Autodesk Inventor part; units mm, degrees
ref_plane "YZ Plane" through (0, 0, 0) normal (1, 0, 0) x (0, 1, 0)
ref_plane "XZ Plane" through (0, 0, 0) normal (0, 1, 0) x (-1, 0, 0)
ref_plane "XY Plane" through (0, 0, 0) normal (0, 0, 1) x (1, 0, 0)
sketch "Sketch1" plane through (0, 0, 0) normal (1, 0, 0) x (0, 1, 0)
  circle A0 centre (0, 0) radius 3.0734
  line L0 (7.62, 7.62) -> (-7.62, 7.62)
  line L1 (-7.62, 7.62) -> (-7.62, -22.86)
  line L2 (-7.62, -22.86) -> (7.62, -22.86)
  line L3 (7.62, -22.86) -> (7.62, 7.62)
  line L4 (-7.62, -22.86) -> (9.652, -22.86)
  line L5 (9.652, -22.86) -> (9.652, -17.78)
  line L6 (9.652, -17.78) -> (-7.62, -17.78)
  line L7 (-7.62, -17.78) -> (-7.62, -22.86)
  line L8 (7.62, -17.78) -> (4.2265, -17.78)
  line L9 (4.2265, -17.78) -> (4.2265, -10.16)
  line L10 (4.2265, -10.16) -> (7.62, -10.16)
  line L11 (7.62, -10.16) -> (7.62, -17.78)
  arc A1 (4.2265, -12.1082) -> (4.2265, -17.78) centre (8.1105, -14.9441) ccw
  line L12 (4.2265, -12.1082) -> (5.6507, -10.16)
  line L13 (4.2265, -17.78) -> (7.62, 0)
  point P0 (7.62, -17.78)
  point P1 (7.62, -22.86)
  point P2 (7.62, -10.16)
  point P3 (7.62, -10.16)
  point P4 (4.2265, -12.1082)
  dimension "d0" = 6.1468
  dimension "d1" = 7.62
  dimension "d2" = 7.62
  dimension "d3" = 7.62
  dimension "d4" = 22.86
  dimension "d5" = 5.08
  dimension "d6" = 2.032
  dimension "d38" = 7.62
extrude "Extrusion1" add sketch "Sketch1" along normal blind 5.334 contours L3 L13 L10 L9 A1 L6 L1 L0 | L6 L3 L2 L1 | L13 L9 L12 L10 | A1 L9 | L6 L5 L4 L3 | L12 L9 L10
sketch "Sketch2" plane through (0, 0, 0) normal (-1, 0, 0) x (0, 0, 1)
  circle A0 centre (0, 0) radius 4.6482
  circle A1 centre (0, 0) radius 10.1706
  dimension "d9" = 9.2964
extrude "Extrusion2" cut sketch "Sketch2" against normal blind 5.334 contours A0
fillet "Fillet1" radius 5.08 3 edges at (2.667, -7.62, -22.86) (2.667, 7.62, 7.62) (2.667, -7.62, 7.62)
sketch "Sketch3" plane through (5.334, 0, 0) normal (1, 0, 0) x (0, 0, -1)
  point P0 (0, 0)
sketch "Sketch7" plane through (0, 0, 0) normal (-1, 0, 0) x (0, 0, 1)
  arc A0 (-2.1195, -5.9858) -> (-2.1254, 5.9838) centre (0, 0) ccw
  line L0 (0, 0) -> (-16.4465, 0)
  arc A1 (-16.4465, 3.175) -> (-17.6024, -2.9571) centre (-16.4465, 0) ccw
  line L1 (-0.2923, 6.3433) -> (-16.4465, 3.175)
  circle A2 centre (-16.4465, 0) radius 3.175
  line L2 (-16.4465, -3.175) -> (-0.2923, -6.3433)
  point P0 (-0.2923, -6.3433)
  point P1 (-17.6024, -2.9571)
  dimension "d33" = 12.7
  dimension "d34" = 16.4465
  dimension "d35" = 6.35
  dimension "d54" = 0
extrude "Extrusion6" cut sketch "Sketch7" against normal blind 2.54 contours L2 A2 L1 A0 | A2 A1
sketch "Sketch8" plane through (2.54, 0, 0) normal (-1, 0, 0) x (0, 0, 1)
  arc A0 (-16.4465, 3.175) -> (-16.4465, -3.175) centre (-16.4465, 0) ccw
  line L0 (0, 0) -> (-16.4465, 0)
  circle A1 centre (-16.4465, 0) radius 1.27
  point P0 (-17.7165, -3.175)
  dimension "d39" = 2.54
  dimension "d46" = 16.4465
extrude "Extrusion7" cut sketch "Sketch8" against normal blind 5.334
sketch "Sketch9" plane through (0, 0, 0) normal (-1, 0, 0) x (0, 0, 1)
  line L0 (2.54, -7.62) -> (-17.78, -7.62)
  line L1 (0, -7.62) -> (-22.6598, -3.952)
  arc A0 (-22.86, -2.54) -> (-17.78, -7.62) centre (-17.78, -2.54) ccw
  point P0 (0, 0)
extrude "Extrusion8" cut sketch "Sketch9" against normal blind 5.334
fillet "Fillet2" radius 3.175 1 edges at (2.667, -3.952, -22.6598)
ref_plane "Work Plane1" through (0, -2.54, 0) normal (0, 0, 1) x (1, 0, 0)
mirror "Mirror1" about plane through (0, -2.54, 0) normal (0, 0, 1) of "Extrusion6"
chamfer "Chamfer3" distance 2.54 distance2 5.08 1 edges at (2.667, 9.652, -17.78) measured on face at (1.778, 9.652, -21.1667)
sketch "Sketch10" plane through (2.54, 0, 0) normal (-1, 0, 0) x (0, 0, 1)
  circle A0 centre (-10.3505, 0) radius 1.27
  circle A1 centre (-16.4465, 0) radius 1.27
  point P0 (0, 0)
  dimension "d50" = 2.54
  dimension "d51" = 6.096
extrude "Extrusion9" cut sketch "Sketch10" against normal blind 5.334 contours A0
sketch "Sketch11" plane through (0, 0, 0) normal (-1, 0, 0) x (0, 0, 1)
  arc A0 (6.9654, 5.0345) -> (2.54, 7.62) centre (2.54, 2.54) ccw
  line L0 (2.54, 7.62) -> (20.32, 4.2879)
  line L1 (20.32, 4.2879) -> (20.32, -4.0399)
  line L2 (20.32, -4.0399) -> (2.54, -7.62)
  arc A1 (2.54, -7.62) -> (6.9654, -5.0345) centre (2.54, -2.54) ccw
  line L3 (0, 13.2262) -> (0, -11.7932)
  line L4 (0, 7.62) -> (2.54, 7.62)
  line L5 (2.54, -7.3934) -> (2.54, -7.62)
  line L6 (2.54, 5.3798) -> (5.1026, 5.3798)
  line L7 (5.1026, 5.3798) -> (5.1026, -5.0345)
  line L8 (5.1026, -5.0345) -> (2.54, -5.0345)
  line L9 (2.54, 7.62) -> (2.54, 5.3798)
  line L10 (2.54, -5.0345) -> (2.54, -7.3934)
  point P0 (0, 0)
  point P1 (2.54, -7.62)
  point P2 (4.5061, -7.2241)
  dimension "d56" = 0
  dimension "d57" = 20.32
extrude "Extrusion10" add sketch "Sketch11" against normal blind 5.334 contours L0 L1 L2 L5 L10 L8 L7 L6 L9
mirror "Mirror2" about plane through (0, -2.54, 0) normal (0, 0, 1) of "Extrusion6", "Extrusion7", "Extrusion9"
fillet "Fillet3" radius 3.175 2 edges at (2.667, 4.2879, 20.32) (2.667, -4.0399, 20.32)
properties part number "ServoHornAdapter"
Work out the finished part from the listing and answer in its coordinate system (mm). A direction names the side the tool comes from. Round coordinates to 2 decimals unless told otherwise and drop trailing zeros. Order: outer loops, then holes, each group sorted by start corner. A loop starts at its lowest first (then second) coordinate and runs counter-clockwise, first axis right, second up. Notation, with made-up numbers: M 55.25,48.25 L 87.25,48.25 A29 ccw 87.25,87.25 Z; hole C 55.5,-19 d1. An arc over 180 degrees is marked long. Put each result on its own line as item: value. Start each with the question number.
Q1. Straight lines are drawn through the part: L1, parallel to X at y = 2.75, z = 8; L2, parallel to Y at x = 4, z = 0; L3, parallel to Z at x = 2.75, y = 0.5. For each, find the intervals that lie inside material, in ascending order. Write a range as [from, to].
Q2. A tool of negligible diameter and unlimited length cuts with its end or side. For faces 5 (the flat face through (3, -7.62, 1)), 6 (the flat face through (2.54, -1, -5)), from which of +Z, -Z, +X, -X, +Y, -Y can it reach the whole face along a straight path? Write none if from no direction.
Q3. Section B-B, the plane z = -10 is taken. Write down the section's boundary in (x, y).
Q4. Section C-C, the plane x = 4.5 is taken. Give the number of separate pieces and of enclosed holes in the cut face, and give its area (3 significant figures).
Q5. Flat-ended cylindrical pins translate along their axes: pin 1 (1.5 mm diameter, centred on y = 0, z = -10.35, fed in from -X); pin 2 (2 mm diameter, centred on x = 4, z = 14, fed in from +Y); pin 3 (3 mm diameter, centred on y = 0, z = 16.45, fed in from -X); pin 4 (2 mm diameter, centred on x = 2.5, z = 2, fed in from +Y). Find the tip coordinate at first contact, or state that the pin passes through.
Q6. Section D-D, the plane z = 7 is taken. Write down the section's boundary in (x, y).
Q7. For a pull along Y with two mould halves and no side action, classify faces 1 (the cylindrical face through (2.704, -7.517, 3.557)), 2 (the flat face through (3, 4, -22.86)), 3 (the flat face through (3, 7.62, 1)), 4 (the cylindrical face through (3.92, 0.49, 9.18)) as pulls with the +Y half, pulls with the -Y half, needs draft (parallel to the pull), parting line crosses it, or undercut.
Q8. Section A-A, the plane y = 0 is taken. Write down the section's boundary in (x, z).
Findings below:
1. L1: x = [2.54, 5.33]
1. L2: y = [-7.62, -4.65], [4.65, 7.62]
1. L3: z = [-22.86, -17.61], [-15.28, -11.52], [-9.18, -4.62], [4.62, 9.18], [11.52, 15.28], [17.61, 20.32]
2. face 5: +Z, -Z, +X, -X, -Y
2. face 6: -X
3. outline: M 0,-6 L 5.33,-6 L 5.33,-1.22 L 2.54,-1.22 L 2.54,-4.44 L 0,-4.44 Z; M 0,4.44 L 2.54,4.44 L 2.54,1.22 L 5.33,1.22 L 5.33,5.71 L 0,5.71 Z
4. separate pieces: 1
4. enclosed holes: 5
4. area: 436 mm^2
5. pin 1: passes through
5. pin 2: stops at y = 5.66
5. pin 3: stops at x = 2.54
5. pin 4: stops at y = 7.62
6. outline: M 0,-6.72 L 5.33,-6.72 L 5.33,6.78 L 0,6.78 L 0,5.03 L 2.54,5.03 L 2.54,-5.03 L 0,-5.03 Z
7. face 1: pulls with the -Y half
7. face 2: needs draft
7. face 3: pulls with the +Y half
7. face 4: undercut
8. outline: M 0,-22.86 L 5.33,-22.86 L 5.33,-17.72 L 2.54,-17.72 L 2.54,-19.62 L 0,-19.62 Z; M 0,19.62 L 2.54,19.62 L 2.54,17.72 L 5.33,17.72 L 5.33,20.32 L 0,20.32 Z; M 2.54,-15.18 L 5.33,-15.18 L 5.33,-11.62 L 2.54,-11.62 Z; M 2.54,-9.08 L 5.33,-9.08 L 5.33,-4.65 L 2.54,-4.65 Z; M 2.54,4.65 L 5.33,4.65 L 5.33,9.08 L 2.54,9.08 Z; M 2.54,11.62 L 5.33,11.62 L 5.33,15.18 L 2.54,15.18 Z
